For this review, take the finished solid that the model builds, in its own axes (mm). A direction names the side the tool comes from. Coordinates: 2 decimals unless noted, no trailing zeros. Write each loop counter-clockwise with the first axis right and the second up, starting at its lowest first coordinate (ties: lowest second). Pieces come first, ordered by that corner, then holes.
```python
from build123d import *

# Parameters (mm, degrees)
SKETCH1_W           = 41.2
SKETCH1_H           = 42
BOSS_EXTRUDE1_DEPTH = 5
CUT_EXTRUDE1_DEPTH  = 3
CUT_EXTRUDE2_DEPTH  = 2
SKETCH6_W           = 5
SKETCH6_H           = 6
BOSS_EXTRUDE2_DEPTH = 5
SKETCH7_W           = 5
SKETCH7_H           = 6
BOSS_EXTRUDE3_DEPTH = 5
SKETCH13_W          = 5
SKETCH13_H          = 6
BOSS_EXTRUDE6_DEPTH = 10
SKETCH10_R          = 1.5
CUT_EXTRUDE3_DEPTH  = 6
FILLET4_R           = 2.5
BOSS_EXTRUDE7_DEPTH = 28
BOSS_EXTRUDE8_DEPTH = 5
FILLET10_R          = 1
FILLET12_R          = 2
FILLET13_R          = 1
FILLET14_R          = 1


with BuildPart() as part:
    # Sketch1 → Boss-Extrude1 (new body)
    with BuildSketch(Plane.XY):
        with Locations((20.6, -21)):
            Rectangle(SKETCH1_W, SKETCH1_H)
    extrude(amount=BOSS_EXTRUDE1_DEPTH)

    # Sketch2 → Cut-Extrude1 (cut)
    with BuildSketch(Plane.XY.offset(5)):
        with BuildLine():
            Line((4, -2), (37.2, -2))
            ThreePointArc((37.2, -2), (38.614213562, -2.585786438), (39.2, -4))
            Line((39.2, -4), (39.2, -38))
            ThreePointArc((39.2, -38), (38.614213562, -39.414213562), (37.2, -40))
            Line((37.2, -40), (4, -40))
            ThreePointArc((4, -40), (2.585786438, -39.414213562), (2, -38))
            Line((2, -38), (2, -4))
            ThreePointArc((2, -4), (2.585786438, -2.585786438), (4, -2))
        make_face()
    extrude(amount=-CUT_EXTRUDE1_DEPTH, mode=Mode.SUBTRACT)

    # Sketch3 → Cut-Extrude2 (cut)
    with BuildSketch(Plane.XY.offset(2)):
        with BuildLine():
            Line((9.25, -7.25), (31.95, -7.25))
            ThreePointArc((31.95, -7.25), (33.364213562, -7.835786438), (33.95, -9.25))
            Line((33.95, -9.25), (33.95, -13.35))
            ThreePointArc((33.95, -13.35), (33.364213562, -14.764213562), (31.95, -15.35))
            Line((31.95, -15.35), (9.25, -15.35))
            ThreePointArc((9.25, -15.35), (7.835786438, -14.764213562), (7.25, -13.35))
            Line((7.25, -13.35), (7.25, -9.25))
            ThreePointArc((7.25, -9.25), (7.835786438, -7.835786438), (9.25, -7.25))
        make_face()
        with BuildLine():
            Line((9.25, -25.85), (31.95, -25.85))
            ThreePointArc((31.95, -25.85), (33.364213562, -26.435786438), (33.95, -27.85))
            Line((33.95, -27.85), (33.95, -32.75))
            ThreePointArc((33.95, -32.75), (33.364213562, -34.164213562), (31.95, -34.75))
            Line((31.95, -34.75), (9.25, -34.75))
            ThreePointArc((9.25, -34.75), (7.835786438, -34.164213562), (7.25, -32.75))
            Line((7.25, -32.75), (7.25, -27.85))
            ThreePointArc((7.25, -27.85), (7.835786438, -26.435786438), (9.25, -25.85))
        make_face()
    extrude(amount=-CUT_EXTRUDE2_DEPTH, mode=Mode.SUBTRACT)

    # Sketch6 → Boss-Extrude2 (add)
    with BuildSketch(Plane(origin=(41.2, 0, 0), x_dir=(0, 0, -1), z_dir=(1, 0, 0))):
        with Locations((-2.5, -31)):
            Rectangle(SKETCH6_W, SKETCH6_H)
    extrude(amount=BOSS_EXTRUDE2_DEPTH)

    # Sketch7 → Boss-Extrude3 (add)
    with BuildSketch(Plane.ZY):
        with Locations((2.5, -31)):
            Rectangle(SKETCH7_W, SKETCH7_H)
    extrude(amount=BOSS_EXTRUDE3_DEPTH)

    # Sketch13 → Boss-Extrude6 (add)
    with BuildSketch(Plane.XY.offset(5)):
        with Locations((43.7, -31)):
            Rectangle(SKETCH13_W, SKETCH13_H)
        with Locations((-2.5, -31)):
            Rectangle(SKETCH13_W, SKETCH13_H)
    extrude(amount=BOSS_EXTRUDE6_DEPTH)

    # Sketch10 → Cut-Extrude3 (cut)
    with BuildSketch(Plane(origin=(0, -28, 0), x_dir=(1, 0, 0), z_dir=(0, 1, 0))):
        with Locations(Location((43.7, -3, 0), (0, 0, 180))):
            Circle(SKETCH10_R)
        with Locations(Location((43.7, -12, 0), (0, 0, 180))):
            Circle(SKETCH10_R)
    cut_extrude3 = extrude(amount=-CUT_EXTRUDE3_DEPTH, mode=Mode.SUBTRACT)

    # Mirror1: Cut-Extrude3 across plane
    add(cut_extrude3.mirror(Plane(origin=(20.6, 0, 0), x_dir=(0, 0, 1), z_dir=(1, 0, 0))), mode=Mode.SUBTRACT)

    # Fillet4
    fillet4_edges = [part.edges().sort_by_distance(p)[0] for p in [
        (-5, -31, 0),
        (46.2, -31, 0),
    ]]
    fillet(fillet4_edges, radius=FILLET4_R)

    # Sketch16 → Boss-Extrude7 (add)
    with BuildSketch(Plane(origin=(0, -28, 0), x_dir=(1, 0, 0), z_dir=(0, 1, 0))):
        with BuildLine():
            Line((41.2, 0), (43.7, 0))
            ThreePointArc((43.7, 0), (45.467766953, -0.732233047), (46.2, -2.5))
            Line((46.2, -2.5), (46.2, -5))
            Line((46.2, -5), (41.2, -5))
            Line((41.2, -5), (41.2, 0))
        make_face()
    boss_extrude7 = extrude(amount=BOSS_EXTRUDE7_DEPTH)

    # Sketch17 → Boss-Extrude8 (add)
    with BuildSketch(Plane(origin=(46.2, 0, 0), x_dir=(0, 0, -1), z_dir=(1, 0, 0))):
        Polygon((-5, 0), (-15, -28), (-5, -28), align=None)
    boss_extrude8 = extrude(amount=-BOSS_EXTRUDE8_DEPTH)

    # Fillet10
    fillet10_edges = [part.edges().sort_by_distance(p)[0] for p in [
        (46.2, -31, 15),
        (46.2, -14, 10),
    ]]
    fillet(fillet10_edges, radius=FILLET10_R)

    # Mirror3: Boss-Extrude7, Boss-Extrude8 across plane
    add(boss_extrude7.mirror(Plane(origin=(20.6, 0, 0), x_dir=(0, 0, 1), z_dir=(1, 0, 0))))
    add(boss_extrude8.mirror(Plane(origin=(20.6, 0, 0), x_dir=(0, 0, 1), z_dir=(1, 0, 0))))

    # Fillet12
    fillet12_edges = [part.edges().sort_by_distance(p)[0] for p in [
        (41.2, -42, 2.5),
        (0, -42, 2.5),
    ]]
    fillet(fillet12_edges, radius=FILLET12_R)

    # Fillet13
    fillet13_edges = [part.edges().sort_by_distance(p)[0] for p in [
        (-5, -31, 15),
        (-5, -14, 10),
    ]]
    fillet(fillet13_edges, radius=FILLET13_R)

    # Fillet14
    fillet14_edges = [part.edges().sort_by_distance(p)[0] for p in [
        (41.2, -17, 5),
        (0, -17, 5),
    ]]
    fillet(fillet14_edges, radius=FILLET14_R)


solid = part.part
```
1) Tool access review of faces 1 (the face through (0, -22, 10)), 2 (the face through (33.35, -26.42, 1.01)), 3 (the face through (38.63, -39.4, 3.52)): name each direction out of +Z, -Z, +X, -X, +Y, -Y from which nothing blocks a thin tool from reaching the whole face with its end or side.
2) Consider section A-A (y = -32). Give the boundary of the cut face in (x, z).
3) The part is to be moulded in two halves that separate along Y. For faces 4 (the face through (40.6, -41.43, 2.54)), 5 (the face through (2.6, -39.43, 3.52)), 6 (the face through (0, -37, 2)), say which applies: pulls with the +Y half, pulls with the -Y half, needs draft (parallel to the pull), parting line crosses it, or undercut.
4) Consider section B-B (x = 10.5). Give the boundary of the cut face in (y, z), then the cut area to 3 significant figures.
5) Clearance check with flat-ended pins moving along their axes: P1, Ø2, axis at x = 2.5, y = -14.5, coming from the +Z side; P2, Ø0.9, axis at x = 44, z = 3, coming from the -Y side; P3, Ø2.5, axis at y = -38.5, z = 3.5, coming from the -X side. State where each tip first meets the part, or that it passes through.
6) For L1, parallel to Y at x = 24.5, z = 1.75; L2, parallel to Z at x = 43.7, y = -32.8; L3, parallel to X at y = -21.5, z = 9, list the stretches that pass through material, from the lowest coordinate up.
Results:
1. face 1: +Z, +Y, -Y
1. face 2: +Z, -Z
1. face 3: +Z
2. outline: (-5, 2.5) arc R2.5 ccw to (-2.5, 0) - (7.25, 0) - (7.25, 2) - (2, 2) - (2, 5) - (1, 5) arc R1 cw to (0, 6) - (0, 15) - (-4, 15) arc R1 ccw to (-5, 14) - close; (33.95, 0) - (43.7, 0) arc R2.5 ccw to (46.2, 2.5) - (46.2, 14) arc R1 ccw to (45.2, 15) - (41.2, 15) - (41.2, 6) arc R1 cw to (40.2, 5) - (39.2, 5) - (39.2, 2) - (33.95, 2) - close; hole circle Ø3 at (-2.5, 3); hole circle Ø3 at (-2.5, 12); hole circle Ø3 at (43.7, 3); hole circle Ø3 at (43.7, 12)
3. face 4: pulls with the -Y half
3. face 5: undercut
3. face 6: needs draft
4. outline: (-42, 0) - (-34.75, 0) - (-34.75, 2) - (-40, 2) - (-40, 5) - (-42, 5) - close; (-25.85, 0) - (-15.35, 0) - (-15.35, 2) - (-25.85, 2) - close; (-7.25, 0) - (0, 0) - (0, 5) - (-2, 5) - (-2, 2) - (-7.25, 2) - close
4. area: 62.0 mm2
5. P1: stops at z = 5
5. P2: stops at y = -28
5. P3: stops at x = 0
6. L1: y = -42 to -34.75, -25.85 to -15.35, -7.25 to 0
6. L2: z = 0 to 1.5, 4.5 to 10.5, 13.5 to 15
6. L3: x = -5 to 0, 41.2 to 46.2
